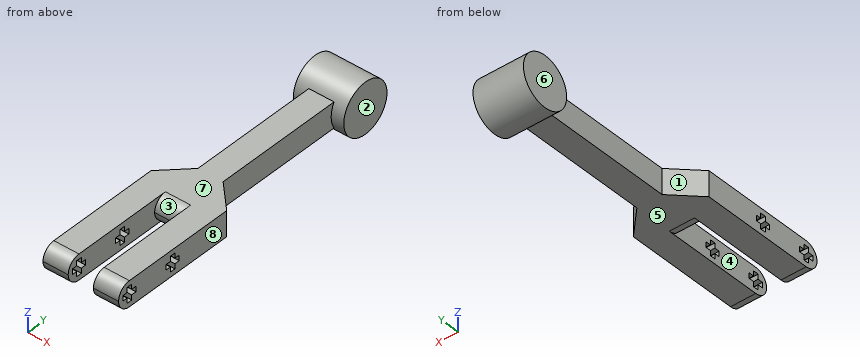
```python
from build123d import *

# Parameters (mm, degrees)
F1_DEPTH     = 7.9375
F2_R         = 3.96874
F3_W         = 1.56845
F3_H         = 1.6891
F3_W_2       = 1.6891
F3_H_2       = 1.56845
F4_DEPTH     = 130
F5_SIZE      = 7.93749
F6_W         = 15.875
F6_H         = 15.875
F7_DEPTH     = 15.875
F8_T1_DEPTH  = 55.5625
F8_T6_DEPTH  = 55.5625
F8_T12_DEPTH = 55.5625
F8_T18_DEPTH = 55.5625
F8_T25_DEPTH = 55.5625
F8_T31_DEPTH = 55.5625
F8_T37_DEPTH = 55.5625
F8_T43_DEPTH = 55.5625
F8_T49_DEPTH = 55.5625
F8_T56_DEPTH = 55.5625
F8_T62_DEPTH = 55.5625


# Not quite as in the source:
# - a fillet or chamfer that OpenCascade refuses, or shapes differently, is made with other operations: its cross-section is extruded or revolved along the edge and cut away or added
# - a fillet or chamfer is up to 0.001 mm smaller than in the source, because OpenCascade refuses the exact size
# - an extrude ends at something that could not be found from the text; its depth is read off the source's solid


with BuildPart() as f1:
    # F0 (on Top) → F1 (new body)
    with BuildSketch(Plane.XY):
        Polygon((0, 39.6875), (0, 0), (7.9375, 0), (7.9375, 31.75), (15.875, 31.75), (15.875, 0), (23.8125, 0), (23.8125, 39.6875), (15.875, 39.6875), (15.875, 87.3125), (7.9375, 87.3125), (7.9375, 39.6875), align=None)
    extrude(amount=F1_DEPTH)

    # F2 (radius 3.96875 in the source; OpenCascade refuses exactly that, so slightly less here)
    f2_edges = [f1.edges().sort_by_distance(p)[0] for p in [
        (3.96875, 0, 0),
        (3.96875, 0, 7.9375),
        (19.84375, 0, 7.9375),
        (19.84375, 0, 0),
        (11.90625, 31.75, 7.9375),
        (11.90625, 31.75, 0),
    ]]
    fillet(f2_edges, radius=F2_R)

    # F3 (on face) → F4 (cut, through all)
    with BuildSketch(Plane(origin=(0, 0, 0), x_dir=(0, -1, 0), z_dir=(-1, 0, 0))):
        with Locations((-2.339975, 3.96875)):
            Rectangle(F3_W, F3_H)
        with Locations((-3.96875, 2.339975)):
            Rectangle(F3_W_2, F3_H_2)
        with Locations((-3.96875, 3.96875)):
            Rectangle(F3_W_2, F3_H)
        with Locations((-5.597525, 3.96875)):
            Rectangle(F3_W, F3_H)
        with Locations((-3.96875, 5.597525)):
            Rectangle(F3_W_2, F3_H_2)
        with Locations((-19.84375, 2.339975)):
            Rectangle(F3_W_2, F3_H_2)
        with Locations((-21.472525, 3.96875)):
            Rectangle(F3_W, F3_H)
        with Locations((-19.84375, 3.96875)):
            Rectangle(F3_W_2, F3_H)
        with Locations((-18.214975, 3.96875)):
            Rectangle(F3_W, F3_H)
        with Locations((-19.84375, 5.597525)):
            Rectangle(F3_W_2, F3_H_2)
    extrude(amount=-F4_DEPTH, mode=Mode.SUBTRACT)

    # F5 (size 7.9375 in the source; OpenCascade refuses exactly that, so slightly less here)
    f5_edges = [f1.edges().sort_by_distance(p)[0] for p in [
        (7.9375, 39.6875, 3.96875),
        (15.875, 39.6875, 3.96875),
    ]]
    chamfer(f5_edges, length=F5_SIZE)

    # F6 (on face) → F7 (join)
    with BuildSketch(Plane(origin=(0, 87.3125, 0), x_dir=(-1, 0, 0), z_dir=(0, 1, 0))):
        with Locations((-11.90625, 3.96875)):
            Rectangle(F6_W, F6_H)
    extrude(amount=F7_DEPTH)

    # F8: fillet of radius 7.9375 on 4 edges, made by hand

    # F8_s2 → F8_t1 (cut)
    with BuildSketch(Plane.YZ.offset(-15.875)):
        with BuildLine():
            ThreePointArc((95.25, -3.96875), (100.8626600757, -1.6439100757), (103.1875, 3.96875))
            Line((103.1875, 3.96875), (103.1875, -3.96875))
            Line((103.1875, -3.96875), (95.25, -3.96875))
        make_face()
        with BuildLine():
            ThreePointArc((95.25, 11.90625), (100.8626600757, 9.5814100757), (103.1875, 3.96875))
            Line((103.1875, 3.96875), (103.1875, 11.90625))
            Line((103.1875, 11.90625), (95.25, 11.90625))
        make_face()
    extrude(amount=F8_T1_DEPTH, mode=Mode.SUBTRACT)


with BuildPart() as f8_tool4:
    # F8_s5 → F8_t6 (new body)
    with BuildSketch(Plane.YZ.offset(39.6875)):
        with BuildLine():
            ThreePointArc((95.25, -3.96875), (89.6373399243, -1.6439100757), (87.3125, 3.96875))
            Line((87.3125, 3.96875), (87.3125, -3.96875))
            Line((87.3125, -3.96875), (95.25, -3.96875))
        make_face()
    extrude(amount=-F8_T6_DEPTH)

    split(bisect_by=Plane.XY, keep=Keep.BOTTOM)

    split(bisect_by=Plane.YZ.offset(15.875), keep=Keep.TOP)


with BuildPart() as f1_1:
    add(f1.part)

    # F8_t3: cut F8_tool4
    add(f8_tool4.part, mode=Mode.SUBTRACT)


with BuildPart() as f8_tool10:
    # F8_s11 → F8_t12 (new body)
    with BuildSketch(Plane.YZ.offset(39.6875)):
        with BuildLine():
            ThreePointArc((95.25, -3.96875), (89.6373399243, -1.6439100757), (87.3125, 3.96875))
            Line((87.3125, 3.96875), (87.3125, -3.96875))
            Line((87.3125, -3.96875), (95.25, -3.96875))
        make_face()
    extrude(amount=-F8_T12_DEPTH)

    split(bisect_by=Plane.XY, keep=Keep.TOP)

    split(bisect_by=Plane.YZ.offset(15.875), keep=Keep.TOP)


with BuildPart() as f1_2:
    add(f1_1.part)

    # F8_t9: cut F8_tool10
    add(f8_tool10.part, mode=Mode.SUBTRACT)


with BuildPart() as f8_tool16:
    # F8_s17 → F8_t18 (new body)
    with BuildSketch(Plane.YZ.offset(39.6875)):
        with BuildLine():
            ThreePointArc((95.25, -3.96875), (89.6373399243, -1.6439100757), (87.3125, 3.96875))
            Line((87.3125, 3.96875), (87.3125, -3.96875))
            Line((87.3125, -3.96875), (95.25, -3.96875))
        make_face()
    extrude(amount=-F8_T18_DEPTH)

    split(bisect_by=Plane.XY, keep=Keep.BOTTOM)

    split(bisect_by=Plane.YZ.offset(7.9375), keep=Keep.TOP)

    split(bisect_by=Plane.YZ.offset(15.875), keep=Keep.BOTTOM)


with BuildPart() as f1_3:
    add(f1_2.part)

    # F8_t15: cut F8_tool16
    add(f8_tool16.part, mode=Mode.SUBTRACT)


with BuildPart() as f8_tool23:
    # F8_s24 → F8_t25 (new body)
    with BuildSketch(Plane.YZ.offset(39.6875)):
        with BuildLine():
            ThreePointArc((95.25, -3.96875), (89.6373399243, -1.6439100757), (87.3125, 3.96875))
            Line((87.3125, 3.96875), (87.3125, -3.96875))
            Line((87.3125, -3.96875), (95.25, -3.96875))
        make_face()
    extrude(amount=-F8_T25_DEPTH)

    split(bisect_by=Plane.XY, keep=Keep.BOTTOM)

    split(bisect_by=Plane.YZ.offset(7.9375), keep=Keep.BOTTOM)


with BuildPart() as f1_4:
    add(f1_3.part)

    # F8_t22: cut F8_tool23
    add(f8_tool23.part, mode=Mode.SUBTRACT)


with BuildPart() as f8_tool29:
    # F8_s30 → F8_t31 (new body)
    with BuildSketch(Plane.YZ.offset(39.6875)):
        with BuildLine():
            ThreePointArc((95.25, -3.96875), (89.6373399243, -1.6439100757), (87.3125, 3.96875))
            Line((87.3125, 3.96875), (87.3125, -3.96875))
            Line((87.3125, -3.96875), (95.25, -3.96875))
        make_face()
    extrude(amount=-F8_T31_DEPTH)

    split(bisect_by=Plane.XY, keep=Keep.TOP)

    split(bisect_by=Plane.YZ.offset(7.9375), keep=Keep.BOTTOM)


with BuildPart() as f1_5:
    add(f1_4.part)

    # F8_t28: cut F8_tool29
    add(f8_tool29.part, mode=Mode.SUBTRACT)


with BuildPart() as f8_tool35:
    # F8_s36 → F8_t37 (new body)
    with BuildSketch(Plane.YZ.offset(-15.875)):
        with BuildLine():
            ThreePointArc((95.25, 11.90625), (89.6373399243, 9.5814100757), (87.3125, 3.96875))
            Line((87.3125, 3.96875), (87.3125, 11.90625))
            Line((87.3125, 11.90625), (95.25, 11.90625))
        make_face()
    extrude(amount=F8_T37_DEPTH)

    split(bisect_by=Plane.YZ.offset(7.9375), keep=Keep.BOTTOM)

    split(bisect_by=Plane.XY.offset(7.9375), keep=Keep.TOP)


with BuildPart() as f1_6:
    add(f1_5.part)

    # F8_t34: cut F8_tool35
    add(f8_tool35.part, mode=Mode.SUBTRACT)


with BuildPart() as f8_tool41:
    # F8_s42 → F8_t43 (new body)
    with BuildSketch(Plane.YZ.offset(-15.875)):
        with BuildLine():
            ThreePointArc((95.25, 11.90625), (89.6373399243, 9.5814100757), (87.3125, 3.96875))
            Line((87.3125, 3.96875), (87.3125, 11.90625))
            Line((87.3125, 11.90625), (95.25, 11.90625))
        make_face()
    extrude(amount=F8_T43_DEPTH)

    split(bisect_by=Plane.YZ.offset(7.9375), keep=Keep.BOTTOM)

    split(bisect_by=Plane.XY.offset(7.9375), keep=Keep.BOTTOM)


with BuildPart() as f1_7:
    add(f1_6.part)

    # F8_t40: cut F8_tool41
    add(f8_tool41.part, mode=Mode.SUBTRACT)


with BuildPart() as f8_tool47:
    # F8_s48 → F8_t49 (new body)
    with BuildSketch(Plane.YZ.offset(-15.875)):
        with BuildLine():
            ThreePointArc((95.25, 11.90625), (89.6373399243, 9.5814100757), (87.3125, 3.96875))
            Line((87.3125, 3.96875), (87.3125, 11.90625))
            Line((87.3125, 11.90625), (95.25, 11.90625))
        make_face()
    extrude(amount=F8_T49_DEPTH)

    split(bisect_by=Plane.YZ.offset(7.9375), keep=Keep.TOP)

    split(bisect_by=Plane.XY.offset(7.9375), keep=Keep.TOP)

    split(bisect_by=Plane.YZ.offset(15.875), keep=Keep.BOTTOM)


with BuildPart() as f1_8:
    add(f1_7.part)

    # F8_t46: cut F8_tool47
    add(f8_tool47.part, mode=Mode.SUBTRACT)


with BuildPart() as f8_tool54:
    # F8_s55 → F8_t56 (new body)
    with BuildSketch(Plane.YZ.offset(-15.875)):
        with BuildLine():
            ThreePointArc((95.25, 11.90625), (89.6373399243, 9.5814100757), (87.3125, 3.96875))
            Line((87.3125, 3.96875), (87.3125, 11.90625))
            Line((87.3125, 11.90625), (95.25, 11.90625))
        make_face()
    extrude(amount=F8_T56_DEPTH)

    split(bisect_by=Plane.XY.offset(7.9375), keep=Keep.TOP)

    split(bisect_by=Plane.YZ.offset(15.875), keep=Keep.TOP)


with BuildPart() as f1_9:
    add(f1_8.part)

    # F8_t53: cut F8_tool54
    add(f8_tool54.part, mode=Mode.SUBTRACT)


with BuildPart() as f8_tool60:
    # F8_s61 → F8_t62 (new body)
    with BuildSketch(Plane.YZ.offset(-15.875)):
        with BuildLine():
            ThreePointArc((95.25, 11.90625), (89.6373399243, 9.5814100757), (87.3125, 3.96875))
            Line((87.3125, 3.96875), (87.3125, 11.90625))
            Line((87.3125, 11.90625), (95.25, 11.90625))
        make_face()
    extrude(amount=F8_T62_DEPTH)

    split(bisect_by=Plane.XY.offset(7.9375), keep=Keep.BOTTOM)

    split(bisect_by=Plane.YZ.offset(15.875), keep=Keep.TOP)


with BuildPart() as f1_10:
    add(f1_9.part)

    # F8_t59: cut F8_tool60
    add(f8_tool60.part, mode=Mode.SUBTRACT)


solid = f1_10.part
```
Input: part model. Units: mm. Frame: model coordinates. Face numbers are marked on the shaded views. A direction names the side the tool comes from. Round coordinates to 2 decimals unless told otherwise and drop trailing zeros. Loops run counter-clockwise (first coordinate to the right, second up) from the corner with the lowest first, then second, coordinate; pieces in that order, holes last. Notation, with made-up numbers: (63, 74) -> (82, 74) arc R14 cw to (82, 87) -> close; hole circle Ø10 at (31.5, -19.75). An arc over 180 degrees is marked (long way). Use one line per item in the form item = value. Start each with the question number.
Item 1: Material intervals for L1, parallel to X at y = 12.5, z = 4.5 (1 decimal); L2, parallel to Y at x = 17, z = 2; L3, parallel to Z at x = 21.25, y = 21.5, sorted ascending. Write a range as from..to.
Item 2: Section query C-C on y = 59. Return the cut outline in (x, z) (1 decimal).
Item 3: Section query A-A on x = 5. Count the separate pieces of the cut face and the enclosed holes in it, then the cut area to 3 significant figures.
Item 4: Contact query for flat-ended pins moving along their axis: pin 1 Ø5 at (x, z) = (17.5, 7.5) entering from +Y; pin 2 Ø1.7 at (x, z) = (21.5, 6) entering from +Y; pin 3 Ø1.9 at (x, y) = (5.5, 20) entering from -Z. Output: stop coordinate, or through.
Item 5: Section query D-D on z = 10.25. Return the cut outline in (x, y), then the cut area to 3 significant figures.
Item 6: Mould query, pull axis X, two halves, no side actions, for the marked faces 1, 2, 3 and 4. Classes: pulls with the +X half, pulls with the -X half, needs draft (parallel to the pull), parting line crosses it, or undercut.
Item 7: Set-up query: the marked faces 5, 6, 7 and 8. Return all of +Z, -Z, +X, -X, +Y, -Y with unobstructed straight access to the full face (end or side cutting, diameter ignored); none if empty.
Ans:
q1.L1 = 0..7.9, 15.9..23.8
q1.L2 = 0.52..3.12, 4.81..19, 20.69..46.5, 87.56..102.94
q1.L3 = 0..3.12, 4.81..7.94
q2.outline = (7.9, 0) -> (15.9, 0) -> (15.9, 7.9) -> (7.9, 7.9) -> close
q3.separate_pieces = 2
q3.enclosed_holes = 2
q3.area = 519 mm^2
q4.pin_1 = 103.12
q4.pin_2 = 42.85
q4.pin_3 = 0
q5.outline = (3.97, 90.4) -> (19.84, 90.4) -> (19.84, 100.1) -> (3.97, 100.1) -> close
q5.area = 154 mm^2
q6.face_1 = pulls with the -X half
q6.face_2 = pulls with the +X half
q6.face_3 = undercut
q6.face_4 = undercut
q7.face_5 = -Z, +X, -X, -Y
q7.face_6 = +Z, -Z, -X, +Y
q7.face_7 = +Z, +X, -X, -Y
q7.face_8 = +Z, -Z, +X, +Y, -Y
